```python
from build123d import *

# Parameters (mm, degrees)
SKETCH3_R           = 2
BOSS_EXTRUDE1_DEPTH = 15
BOSS_EXTRUDE2_DEPTH = 1
SKETCH6_R           = 3.5
BOSS_EXTRUDE3_DEPTH = 11
SKETCH7_R           = 2
BOSS_EXTRUDE4_DEPTH = 9
CHAMFER2_SIZE       = 0.5
SKETCH9_R           = 2
BOSS_EXTRUDE5_DEPTH = 7


with BuildPart() as part:
    # Sketch2 → Revolve1 (revolve)
    with BuildSketch(Plane(origin=(0, 0, 0), x_dir=(0, 0, -1), z_dir=(1, 0, 0)), mode=Mode.PRIVATE) as revolve1_sk:
        Polygon((0, 0), (0, 22), (-4, 16), (-4, 0), align=None)
    revolve(revolve1_sk.sketch.rotate(Axis((0, 0, 4), (0, 0, -1)), 90), axis=Axis((0, 0, 4), (0, 0, -1)))

    # Sketch3 → Boss-Extrude1 (add)
    with BuildSketch(Plane.XY.offset(4)):
        with Locations(Location((7.94445625, -4.586733955, 0), (0, 0, 180))):
            Circle(SKETCH3_R)
        with Locations(Location((-7.94445625, -4.586733955, 0), (0, 0, 180))):
            Circle(SKETCH3_R)
        with Locations(Location((0, 9.173467909, 0), (0, 0, 180))):
            Circle(SKETCH3_R)
    extrude(amount=BOSS_EXTRUDE1_DEPTH)

    # Sketch4 → Boss-Extrude2 (add)
    with BuildSketch(Plane.XY.offset(19)):
        with BuildLine():
            Line((1.732050808, 10.173467909), (9.676507058, -3.586733955))
            ThreePointArc((9.676507058, -3.586733955), (9.676507058, -5.586733955), (7.94445625, -6.586733955))
            Line((7.94445625, -6.586733955), (-7.94445625, -6.586733955))
            ThreePointArc((-7.94445625, -6.586733955), (-9.676507058, -5.586733955), (-9.676507058, -3.586733955))
            Line((-9.676507058, -3.586733955), (-1.732050808, 10.173467909))
            ThreePointArc((-1.732050808, 10.173467909), (0, 11.173467909), (1.732050808, 10.173467909))
        make_face()
    extrude(amount=BOSS_EXTRUDE2_DEPTH)

    # Sketch6 → Boss-Extrude3 (add)
    with BuildSketch(Plane.XY.offset(20)):
        Circle(SKETCH6_R)
    extrude(amount=BOSS_EXTRUDE3_DEPTH)

    # Sketch7 → Boss-Extrude4 (add)
    with BuildSketch(Plane.XY.offset(31)):
        Circle(SKETCH7_R)
    extrude(amount=BOSS_EXTRUDE4_DEPTH)

    # Chamfer2
    chamfer2_edges = [part.edges().sort_by_distance(p)[0] for p in [
        (-3.5, 0, 31),
    ]]
    chamfer(chamfer2_edges, length=CHAMFER2_SIZE)

    # Sketch8 → Revolve2 (revolve)
    with BuildSketch(Plane(origin=(0, 0, 0), x_dir=(1, 0, 0), z_dir=(0, 1, 0)), mode=Mode.PRIVATE) as revolve2_sk:
        with BuildLine():
            Line((0, -40), (2, -40))
            ThreePointArc((2, -40), (4.985127596, -41.278519641), (6.191881653, -44.293373514))
            Line((6.191881653, -44.293373514), (6.861274265, -44.293373514))
            Line((6.861274265, -44.293373514), (6.861274265, -45.241679714))
            Line((6.861274265, -45.241679714), (5.57827176, -45.241679714))
            ThreePointArc((5.57827176, -45.241679714), (4.736480165, -42.213503946), (2, -40.66749687))
            Line((2, -40.66749687), (0, -40.66749687))
            Line((0, -40.66749687), (0, -40))
        make_face()
    revolve(revolve2_sk.sketch.rotate(Axis((0, 0, 40), (0, 0, 1)), 180), axis=Axis((0, 0, 40), (0, 0, 1)))

    # Sketch9 → Boss-Extrude5 (add)
    with BuildSketch(Plane(origin=(0, 0, 0), x_dir=(0, 0, -1), z_dir=(1, 0, 0))):
        with Locations((-25.382084378, 0)):
            Circle(SKETCH9_R)
    extrude(amount=-BOSS_EXTRUDE5_DEPTH)


solid = part.part
```
Build history of the part. All positions in model axes, mm. A direction names the side the tool comes from. Give positions to 0.01 mm unless a question says otherwise; leave off trailing zeros. Loops run counter-clockwise (first coordinate to the right, second up) from the corner with the lowest first, then second, coordinate; pieces in that order, holes last. Notation, with made-up numbers: (19, -26) - (37, -26) arc R26 cw to (37, -2) - close; hole circle Ø3 at (53.25, 33). An arc over 180 degrees is marked (long way). Use a Markdown table: item, result.
(1) Pull direction X, two halves, no side cores. Call faces 1 (the face through (-4.907, -0.766, 23.535)), 2 (the face through (0, 0, 40.667)), 3 (the face through (3.34, 1.05, 25.18)): +X half, -X half, draft (parallel to the pull), parting line (faces both ways), or undercut.
Taken from the geometry:
| item | result |
|---|---|
| face 1 | draft |
| face 2 | undercut |
| face 3 | parting line |
(2) Wall check: line 1 along Z through (x, y) = (3, 1); line 2 along Z through (x, y) = (-5, 6.5); line 3 along X through (y, z) = (-4, 8). Give the ranges that are in metal, low to high.
Taken from the geometry:
| item | result |
|---|---|
| line 1 | 0 to 4, 19 to 30.84, 40.18 to 40.99 |
| line 2 | 0 to 4 |
| line 3 | -9.86 to -6.03, 6.03 to 9.86 |
(3) Band-saw the part on B-B (z = 12). Give the cut face in (x, y).
Taken from the geometry:
| item | result |
|---|---|
| outline | circle Ø4 at (-7.94, -4.59); circle Ø4 at (0, 9.17); circle Ø4 at (7.94, -4.59) |
(4) Which spindle directions (+Z, -Z, +X, -X, +Y, -Y) get a long thin tool onto all of the face, cutting with end or side? Do faces 4 (the face through (-3.166, 6.087, 44.774)), 5 (the face through (-7, 0, 25)), 6 (the face through (-5.76, 3.2, 19.49)), 7 (the face through (-4, -5, 44.293)). Say none if no direction does.
Taken from the geometry:
| item | result |
|---|---|
| face 4 | +Z |
| face 5 | +Z, -X, +Y, -Y |
| face 6 | -X, +Y |
| face 7 | none |
(5) Band-saw the part on A-A (z = 35). Give the cut face in (x, y).
Taken from the geometry:
| item | result |
|---|---|
| outline | circle Ø4 at (0, 0) |
(6) Drop flat-ended pins along their axis: pin 1 Ø6.5 at (x, y) = (-1.5, 0) entering from +Z; pin 2 Ø5 at (x, y) = (-13.5, 14) entering from +Z; pin 3 Ø1.2 at (x, y) = (1, 0) entering from +Z. Give the stop position or say it passes through.
Taken from the geometry:
| item | result |
|---|---|
| pin 1 | z = 42.23 |
| pin 2 | z = 3.37 |
| pin 3 | z = 40.67 |
